Design review of the part built by this model. Coordinates are the model's own, in mm. Face numbers are marked on the shaded views. A direction names the side the tool comes from. Round coordinates to 2 decimals unless told otherwise and drop trailing zeros. Loops run counter-clockwise (first coordinate to the right, second up) from the corner with the lowest first, then second, coordinate; pieces in that order, holes last. Notation, with made-up numbers: (20.5, -7) - (71.5, -7) arc R22 ccw to (71.5, 2) - close; hole circle Ø11 at (58.25, -14). An arc over 180 degrees is marked (long way). Return JSON: item names as keys, results as strings. Group by question number.
from build123d import *

# Parameters (mm, degrees)
SKETCH5_R           = 13
BOSS_EXTRUDE3_DEPTH = 3.5
SKETCH6_W           = 6.5
SKETCH6_H           = 20
BOSS_EXTRUDE4_DEPTH = 3.5
SKETCH9_R           = 1.75
CUT_EXTRUDE1_DEPTH  = 3.5
FILLET1_R           = 2
BOSS_EXTRUDE5_DEPTH = 3.5


with BuildPart() as part:
    # Sketch5 → Boss-Extrude3 (new body)
    with BuildSketch(Plane.XY.offset(3)):
        with Locations((0, 20.92523633)):
            Circle(SKETCH5_R)
    extrude(amount=BOSS_EXTRUDE3_DEPTH)

    # Sketch6 → Boss-Extrude4 (add)
    with BuildSketch(Plane.XY.offset(3)):
        with Locations((0.239986303, 43.081718219)):
            Rectangle(SKETCH6_W, SKETCH6_H)
    extrude(amount=BOSS_EXTRUDE4_DEPTH)

    # Sketch9 → Cut-Extrude1 (cut)
    with BuildSketch(Plane(origin=(0, 0, 3), x_dir=(-1, 0, 0), z_dir=(0, 0, -1))):
        with Locations((-0.239986303, 49.531718219)):
            Circle(SKETCH9_R)
        with Locations((-0.239986303, 20.92523633)):
            Circle(SKETCH9_R)
    extrude(amount=-CUT_EXTRUDE1_DEPTH, mode=Mode.SUBTRACT)

    # Fillet1
    fillet1_edges = [part.edges().sort_by_distance(p)[0] for p in [
        (-3.010013697, 53.081718219, 4.75),
        (3.489986303, 53.081718219, 4.75),
    ]]
    fillet(fillet1_edges, radius=FILLET1_R)

    # Sketch10 → Boss-Extrude5 (add)
    with BuildSketch(Plane.XY.offset(3)):
        with BuildLine():
            Line((-5.759354429, 32.464504571), (-3.919377514, 33.177547189))
            ThreePointArc((-3.919377514, 33.177547189), (-4.520656892, 34.95869799), (-6.174793625, 35.851931857))
            ThreePointArc((-6.174793625, 35.851931857), (-6.596620884, 34.081009637), (-5.759354429, 32.464504571))
        make_face()
        with BuildLine():
            Line((-8.258779816, 30.769918915), (-6.632838661, 31.888069256))
            ThreePointArc((-6.632838661, 31.888069256), (-7.628672119, 33.482544339), (-9.444215288, 33.970230789))
            ThreePointArc((-9.444215288, 33.970230789), (-9.446269369, 32.149763946), (-8.258779816, 30.769918915))
        make_face()
        with BuildLine():
            Line((-10.300034522, 28.544603873), (-8.975784035, 30.007582162))
            ThreePointArc((-8.975784035, 30.007582162), (-10.312485934, 31.329422963), (-12.191559136, 31.385270693))
            ThreePointArc((-12.191559136, 31.385270693), (-11.773729303, 29.613401065), (-10.300034522, 28.544603873))
        make_face()
        with BuildLine():
            Line((-11.773073977, 25.908526755), (-10.821904846, 27.637463454))
            ThreePointArc((-10.821904846, 27.637463454), (-12.427413239, 28.615409193), (-14.268715153, 28.236407437))
            ThreePointArc((-14.268715153, 28.236407437), (-13.45352672, 26.608656975), (-11.773073977, 25.908526755))
        make_face()
        with BuildLine():
            Line((-12.598486243, 23.00379916), (-12.071676241, 24.905486844))
            ThreePointArc((-12.071676241, 24.905486844), (-13.859437756, 25.486816213), (-15.563703318, 24.693397054))
            ThreePointArc((-15.563703318, 24.693397054), (-14.395103305, 23.297518207), (-12.598486243, 23.00379916))
        make_face()
        with BuildLine():
            Line((-12.731773131, 19.987015705), (-12.657722722, 21.958933898))
            ThreePointArc((-12.657722722, 21.958933898), (-14.531358672, 22.11230728), (-16.006710485, 20.947244151))
            ThreePointArc((-16.006710485, 20.947244151), (-14.547698421, 19.858489109), (-12.731773131, 19.987015705))
        make_face()
        with BuildLine():
            Line((-12.16574911, 17.020811966), (-12.54845037, 18.956654049))
            ThreePointArc((-12.54845037, 18.956654049), (-14.406952557, 18.673803046), (-15.573854024, 17.199904801))
            ThreePointArc((-15.573854024, 17.199904801), (-13.903085626, 16.476968629), (-12.16574911, 17.020811966))
        make_face()
        with BuildLine():
            Line((-10.930928682, 14.265096756), (-11.749750088, 16.060500981))
            ThreePointArc((-11.749750088, 16.060500981), (-13.492926178, 15.356674163), (-14.288469337, 13.653399038))
            ThreePointArc((-14.288469337, 13.653399038), (-12.496016163, 13.335255413), (-10.930928682, 14.265096756))
        make_face()
        with BuildLine():
            Line((-9.093881336, 11.868431394), (-10.304680013, 13.426607054))
            ThreePointArc((-10.304680013, 13.426607054), (-11.838554931, 12.339747907), (-12.219851845, 10.498919905))
            ThreePointArc((-12.219851845, 10.498919905), (-10.40234551, 10.602720033), (-9.093881336, 11.868431394))
        make_face()
        with BuildLine():
            Line((-6.753642769, 9.96002073), (-8.291144248, 11.196966172))
            ThreePointArc((-8.291144248, 11.196966172), (-9.533026401, 9.785667555), (-9.479521255, 7.90652619))
            ThreePointArc((-9.479521255, 7.90652619), (-7.734943995, 8.426674178), (-6.753642769, 9.96002073))
        make_face()
        with BuildLine():
            Line((-4.036375849, 8.642747678), (-5.817693027, 9.491778853))
            ThreePointArc((-5.817693027, 9.491778853), (-6.700632226, 7.832124238), (-6.215209496, 6.015974508))
            ThreePointArc((-6.215209496, 6.015974508), (-4.637611923, 6.924429043), (-4.036375849, 8.642747678))
        make_face()
        with BuildLine():
            Line((-1.088569138, 7.987626768), (-3.017670745, 8.402972186))
            ThreePointArc((-3.017670745, 8.402972186), (-3.494067509, 6.584433984), (-2.60289646, 4.92918499))
            ThreePointArc((-2.60289646, 4.92918499), (-1.277327268, 6.176971054), (-1.088569138, 7.987626768))
        make_face()
        with BuildLine():
            Line((1.93086034, 8.029975738), (-0.042027328, 7.98924402))
            ThreePointArc((-0.042027328, 7.98924402), (-0.086198985, 6.109860096), (1.162677121, 4.704746741))
            ThreePointArc((1.162677121, 4.704746741), (2.164756155, 6.224595863), (1.93086034, 8.029975738))
        make_face()
    extrude(amount=BOSS_EXTRUDE5_DEPTH)


solid = part.part
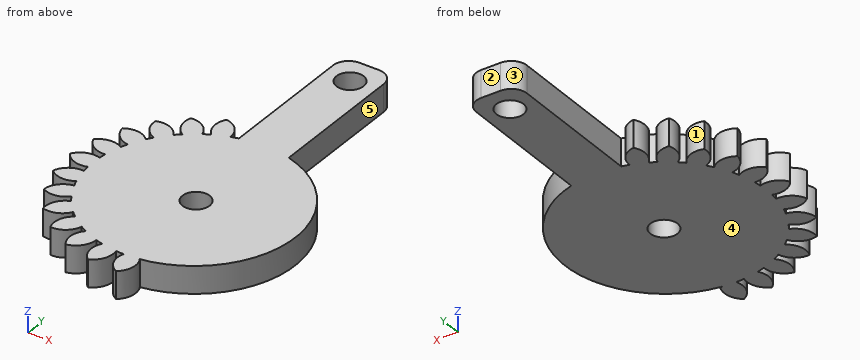
Q1. Add section C-C, the plane x = 6. State the section outline as (y, z) points.
Q2. Add section B-B, the plane z = 5.75. Give the number of separate pieces and of enclosed holes in the cut face, plus the area to 3 significant figures.
Q3. Add section A-A, the plane y = 45. State the section outline as (x, z) points, plus the area to 4 significant figures.
Q4. Draft analysis for pull direction X (two halves, no side actions). For the marked faces 1, 2 and 3, state which applies: pulls with the +X half, pulls with the -X half, needs draft (parallel to the pull), parting line crosses it, or undercut.
Q5. For line 1 (X direction, y = 39.5, z = 6.2); line 2 (Y direction, x = -14, z = 3.65); line 3 (X direction, y = 21.5, z = 3.35), list the stretches that pass through material, from the lowest coordinate up.
Q6. Insertion check: pin 1 Ø1 at (x, z) = (0, 5.5) entering from -Y; pin 2 Ø2 at (y, z) = (46.5, 4) entering from -X; pin 3 Ø1 at (x, z) = (-13, 5.5) entering from +Y. Each pin has a flat end and moves straight along its axis. Give the tip position at first contact, or say it passes through.
Q7. Tool access review of the marked faces 4 and 5: name each direction out of +Z, -Z, +X, -X, +Y, -Y from which nothing blocks a thin tool from reaching the whole face with its end or side.
Evaluation:
{
 "1": {"outline": "(9.39, 3) - (32.46, 3) - (32.46, 6.5) - (9.39, 6.5) - close"},
 "2": {"separate pieces": "1", "enclosed holes": "2", "area": "713 mm²"},
 "3": {"outline": "(-3.01, 3) - (3.49, 3) - (3.49, 6.5) - (-3.01, 6.5) - close", "area": "22.75 mm²"},
 "4": {"face 1": "undercut", "face 2": "needs draft", "face 3": "pulls with the -X half"},
 "5": {"line 1": "-3.01 to 3.49", "line 2": "13.51 to 14.69, 16.48 to 18.86, 19.76 to 22.21, 23.11 to 25.47, 27.33 to 28.39", "line 3": "-15.57 to -1.41, 1.89 to 12.99"},
 "6": {"pin 1": "y = 5.19", "pin 2": "x = -3.01", "pin 3": "y = 28.65"},
 "7": {"face 4": "-Z, +X, -X, +Y, -Y", "face 5": "+Z, -Z, +X, +Y"}
}
